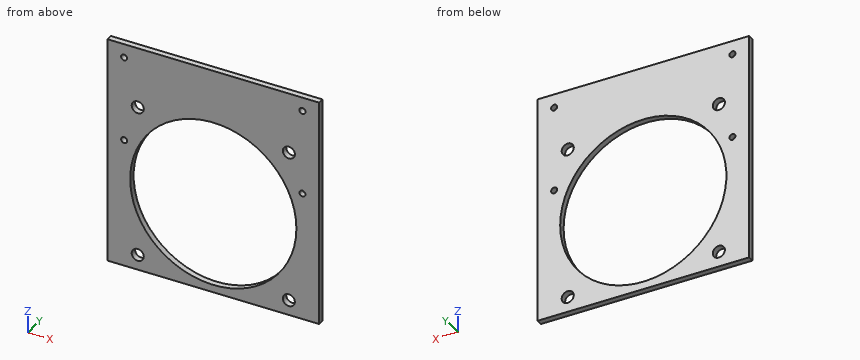
Autodesk Inventor part; units mm, degrees
ref_plane "YZ Plane" through (0, 0, 0) normal (1, 0, 0) x (0, 1, 0)
ref_plane "XZ Plane" through (0, 0, 0) normal (0, 1, 0) x (-1, 0, 0)
ref_plane "XY Plane" through (0, 0, 0) normal (0, 0, 1) x (1, 0, 0)
sketch "Sketch1" plane through (0, 0, 0) normal (0, 1, 0) x (-1, 0, 0)
  line L0 (0, 0) -> (-70, 0)
  line L1 (-70, 0) -> (-70, 75)
  line L2 (-70, 75) -> (0, 75)
  line L3 (0, 75) -> (0, 0)
  dimension "d0" = 75
  dimension "d1" = 70
extrude "Extrusion1" add sketch "Sketch1" along normal blind 2
sketch "Sketch2" plane through (0, 0, 0) normal (0, -1, 0) x (1, 0, 0)
  line L0 (70, 0) -> (70, 75)
  line L1 (70, 75) -> (0, 75)
  circle A0 centre (60, 55) radius 2
  circle A1 centre (10, 55) radius 2
  circle A2 centre (60, 5) radius 2
  circle A3 centre (10, 5) radius 2
  line L2 (0, 0) -> (70, 0)
  line L3 (35, 75) -> (35, 0) construction
  line L4 (5, 0) -> (65, 0) construction
  line L5 (65, 0) -> (65, 60) construction
  line L6 (65, 60) -> (5, 60) construction
  line L7 (5, 60) -> (5, 0) construction
  line L8 (5, 0) -> (65, 60) construction
  line L9 (65, 0) -> (5, 60) construction
  circle A4 centre (35, 30) radius 27.5
  dimension "d7" = 4
  dimension "d44" = 50
  dimension "d47" = 50
  dimension "d56" = 55
  dimension "d71" = 60
  dimension "d72" = 60
  dimension "d73" = 30
  dimension "d74" = 5
  dimension "d75" = 55
extrude "Extrusion2" cut sketch "Sketch2" against normal through all
sketch "Sketch5" plane through (0, 0, 0) normal (0, -1, 0) x (1, 0, 0)
  line L0 (0, 0) -> (70, 0)
  line L1 (70, 0) -> (70, 75)
  line L2 (70, 75) -> (0, 75)
  circle A0 centre (64.5, 70.5) radius 1
  circle A1 centre (5.5, 70.5) radius 1
  circle A2 centre (64.5, 42.5) radius 1
  circle A3 centre (5.5, 42.5) radius 1
  line L3 (35, 75) -> (35, 0) construction
  dimension "d57" = 2
  dimension "d58" = 4.5
  dimension "d61" = 59
  dimension "d64" = 28
  dimension "d68" = 59
extrude "Extrusion5" cut sketch "Sketch5" against normal through all
properties part number "base_usb3"
Geometry: final body of the model. Coordinates: model frame, mm. Round coordinates to 2 decimals unless told otherwise and drop trailing zeros. Write each loop counter-clockwise with the first axis right and the second up, starting at its lowest first coordinate (ties: lowest second). Pieces come first, ordered by that corner, then holes. Notation, with made-up numbers: M -24.5,8 L 20.5,8 A5 cw 20.5,17 Z; hole C 68,-15 d4. An arc over 180 degrees is marked long. Write item = value, one per line.
Item 1: Section query B-B on x = 35. Return loops of the section in (y, z), then the cut area to 3 significant figures.
Findings:
outline = M 0,0 L 2,0 L 2,2.5 L 0,2.5 Z; M 0,57.5 L 2,57.5 L 2,75 L 0,75 Z
area = 40.0 mm^2
Item 2: Section query C-C on z = 16. Return loops of the section in (x, y), then the cut area to 3 significant figures.
Findings:
outline = M 0,0 L 11.33,0 L 11.33,2 L 0,2 Z; M 58.67,0 L 70,0 L 70,2 L 58.67,2 Z
area = 45.3 mm^2
Item 3: Section query A-A on z = 70.5. Return loops of the section in (x, y), then the cut area to 3 significant figures.
Findings:
outline = M 0,0 L 4.5,0 L 4.5,2 L 0,2 Z; M 6.5,0 L 63.5,0 L 63.5,2 L 6.5,2 Z; M 65.5,0 L 70,0 L 70,2 L 65.5,2 Z
area = 132 mm^2
Item 4: Section query D-D on y = 1.65. State how many separate pieces and enclosed holes the cut face has, then the cut area to 3 significant figures.
Findings:
separate_pieces = 1
enclosed_holes = 9
area = 2,810 mm^2
Item 5: Material intervals for line 1 along Z through (x, y) = (5.5, 0.8); line 2 along X through (y, z) = (1.55, 70.5); line 3 along Z through (x, y) = (60, 0.95), sorted ascending. Write a range as [from, to].
Findings:
line_1 = [0, 41.5], [43.5, 69.5], [71.5, 75]
line_2 = [0, 4.5], [6.5, 63.5], [65.5, 70]
line_3 = [0, 3], [7, 18.54], [41.46, 53], [57, 75]
Item 6: Pin query (flat end, axial travel): P1, Ø3, axis at x = 10, z = 55, coming from the +Y side; P2, Ø2.5, axis at x = 5.5, z = 42.5, coming from the -Y side. Return the tip coordinate at first contact, or that it passes through.
Findings:
P1 = through
P2 = 0
